Input: part model. Units: mm. Frame: model coordinates. Face numbers are marked on the shaded views. Coordinates: 2 decimals unless noted, no trailing zeros. Loops run counter-clockwise (first coordinate to the right, second up) from the corner with the lowest first, then second, coordinate; pieces in that order, holes last. Notation, with made-up numbers: (72, -28) -> (99, -28) arc R10 cw to (99, -10) -> close; hole circle Ø6 at (59.5, 76.25). An arc over 180 degrees is marked (long way). Answer as a JSON object with one key per item and string values.
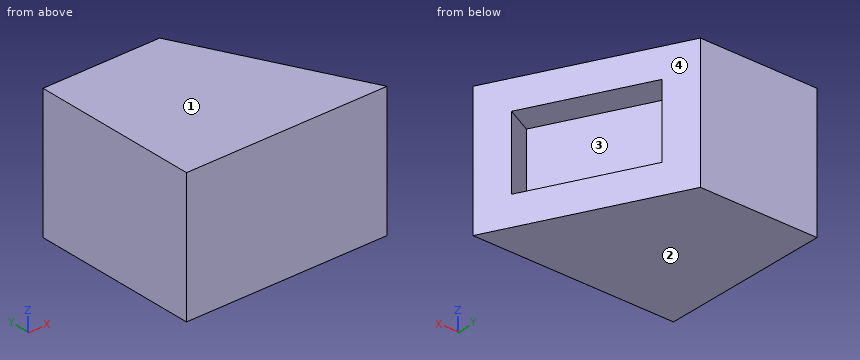
from build123d import *

# Parameters (mm, degrees)
BOSS_EXTRUDE1_DEPTH = 180
SKETCH3_W           = 100
SKETCH3_H           = 170
CUT_EXTRUDE4_DEPTH  = 50


with BuildPart() as part:
    # Sketch1 → Boss-Extrude1 (new body)
    with BuildSketch(Plane.XY):
        Polygon((0, 0), (275, 0), (160, 230), (0, 230), align=None)
    extrude(amount=-BOSS_EXTRUDE1_DEPTH)

    # Sketch3 → Cut-Extrude4 (cut)
    with BuildSketch(Plane(origin=(228.94427191, 114.472135955, 0), x_dir=(0, 0, -1), z_dir=(0.894427191, 0.447213595, 0))):
        with Locations((90, 5.590169944)):
            Rectangle(SKETCH3_W, SKETCH3_H)
    extrude(amount=-CUT_EXTRUDE4_DEPTH, mode=Mode.SUBTRACT)


solid = part.part
1. Mould query, pull axis Z, two halves, no side actions, for the marked faces 1, 2, 3 and 4. Classes: pulls with the +Z half, pulls with the -Z half, needs draft (parallel to the pull), parting line crosses it, or undercut.
Reply:
{"face 1": "pulls with the +Z half", "face 2": "pulls with the -Z half", "face 3": "undercut", "face 4": "needs draft"}
2. Section query D-D (y = 203). Return loops of the section in (x, z).
Reply:
{"outline": "(0, -180) -> (173.5, -180) -> (173.5, 0) -> (0, 0) -> close"}
3. Line query: line 1 along Z through (x, y) = (180, 151.5); line 2 along Y through (x, z) = (150, -69); line 3 along X through (y, z) = (90, -14.5). Output: solid intervals per line, ascending.
Reply:
{"line 1": "z = -180 to -140, -40 to 0", "line 2": "y = 0 to 160.56, 176.28 to 230", "line 3": "x = 0 to 230"}
4. Section query A-A (x = 167). Return loops of the section in (y, z), plus the area to 3 significant figures.
Reply:
{"outline": "(0, -180) -> (216, -180) -> (216, 0) -> (0, 0) -> close; hole (126.56, -140) -> (184.78, -140) -> (184.78, -40) -> (126.56, -40) -> close", "area": "33,100 mm2"}
5. Section query B-B (y = 51). Return loops of the section in (x, z), plus the area to 3 significant figures.
Reply:
{"outline": "(0, -180) -> (249.5, -180) -> (249.5, -140) -> (204.78, -140) -> (204.78, -40) -> (249.5, -40) -> (249.5, 0) -> (0, 0) -> close", "area": "40,400 mm2"}
6. Section query C-C (z = -123.5). Return loops of the section in (x, y), plus the area to 3 significant figures.
Reply:
{"outline": "(0, 0) -> (275, 0) -> (255.51, 38.97) -> (219.74, 21.09) -> (143.71, 173.14) -> (179.49, 191.03) -> (160, 230) -> (0, 230) -> close", "area": "43,200 mm2"}
